The model under review builds one solid part; all positions refer to its coordinate system, in mm. Face numbers are marked on the shaded views. A direction names the side the tool comes from. Coordinates: 2 decimals unless noted, no trailing zeros. Loops run counter-clockwise (first coordinate to the right, second up) from the corner with the lowest first, then second, coordinate; pieces in that order, holes last. Notation, with made-up numbers: M 66,65 L 84,65 A36 ccw 84,103 Z; hole C 36.5,15 d11. An arc over 180 degrees is marked long. Use CSV: the item, a comma, the result in double quotes. Start each with the question number.
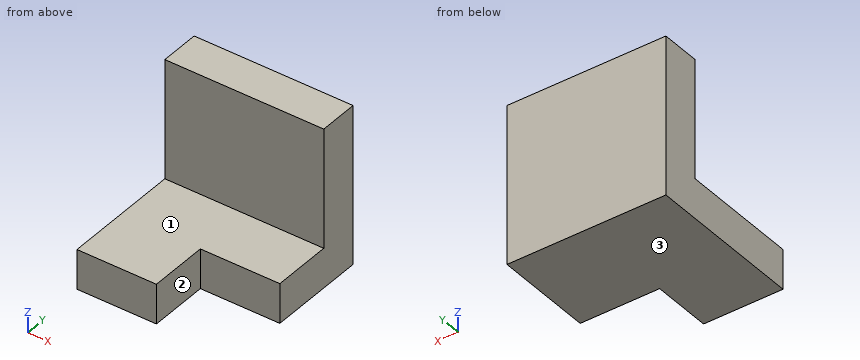
from build123d import *

# Parameters (mm, degrees)
F0_W     = 100
F0_H     = 100
F1_DEPTH = 100
F2_W     = 100
F2_H     = 75
F3_DEPTH = 75
F4_W     = 50
F4_H     = 37.5
F5_DEPTH = 25.001


with BuildPart() as f1:
    # F0 (on Top) → F1 (new body)
    with BuildSketch(Plane.XY):
        with Locations((-50, 50)):
            Rectangle(F0_W, F0_H)
    extrude(amount=-F1_DEPTH)

    # F2 (on face) → F3 (cut)
    with BuildSketch(Plane.XY):
        with Locations((-50, 37.5)):
            Rectangle(F2_W, F2_H)
    extrude(amount=-F3_DEPTH, mode=Mode.SUBTRACT)

    # F4 (on face) → F5 (cut, through all)
    with BuildSketch(Plane.XY.offset(-75)):
        with Locations((-25, 18.75)):
            Rectangle(F4_W, F4_H)
    extrude(amount=-F5_DEPTH, mode=Mode.SUBTRACT)


solid = f1.part
1. For the marked faces 1, 2 and 3, list the 3-axis set-ups (+Z, -Z, +X, -X, +Y, -Y) from which the entire face can be reached by the end or side of a thin tool; tool diameter is ignored.
2. To check wall thickness, follow line 1 along Z through (x, y) = (-10.5, 48); line 2 along Y through (x, z) = (-25, -74); line 3 along Y through (x, z) = (-38, -87.5). State the ranges of each line that lie inside material, in increasing order.
3. Add section B-B (x = -52.5). Write out the cut boundary in (y, z).
4. Add section A-A (z = -82.5). Write out the cut boundary in (x, y), plus the area to 4 significant figures.
5. Add section D-D (z = -59). Write out the cut boundary in (x, y), plus the area to 3 significant figures.
6. Add section C-C (y = 34.5). Write out the cut boundary in (x, z).
7. Insertion check: pin 1 Ø2 at (x, y) = (-88.5, 41.5) entering from +Z; pin 2 Ø22.5 at (x, z) = (-39.5, -50) entering from -Y; pin 3 Ø7.5 at (y, z) = (22, -89.5) entering from +X. Each pin has a flat end and moves straight along its axis. Give the tip position at first contact, or say it passes through.
Solved:
1,face 1,"+Z, +X, -X, -Y"
1,face 2,"+Z, -Z, +X, -Y"
1,face 3,"-Z, +X, -X, +Y, -Y"
2,line 1,"z = -100 to -75"
2,line 2,"y = 75 to 100"
2,line 3,"y = 37.5 to 100"
3,outline,"M 0,-100 L 100,-100 L 100,0 L 75,0 L 75,-75 L 0,-75 Z"
4,outline,"M -100,0 L -50,0 L -50,37.5 L 0,37.5 L 0,100 L -100,100 Z"
4,area,"8,125 mm^2"
5,outline,"M -100,75 L 0,75 L 0,100 L -100,100 Z"
5,area,"2,500 mm^2"
6,outline,"M -100,-100 L -50,-100 L -50,-75 L -100,-75 Z"
7,pin 1,"stops at z = -75"
7,pin 2,"stops at y = 75"
7,pin 3,"stops at x = -50"
